```python
from build123d import *

# Parameters (mm, degrees)
ESQUISSE4_R                = 1.3
FIXINGHOLE_DEPTH           = 35
FIXINGHOLEREPETITION_COUNT = 8
RIGHTFIXING_DEPTH          = 10
ESQUISSE7_R                = 1.6
TOPFIXINGHOLES_DEPTH       = 8.6
HOLEFORFIXING_DEPTH        = 51


with BuildPart() as part:
    # Esquisse1 → Révolution1 (revolve)
    with BuildSketch(Plane.XY):
        Polygon((14, 0), (14, 34), (19, 34), (19, 5), (24, 5), (24, 0), align=None)
    revolve(axis=Axis((0, -1.825, 0), (0, 1, 0)))

    # Esquisse4 → FixingHole (cut, through all)
    with BuildSketch(Plane(origin=(0, 0, 0), x_dir=(-1, 0, 0), z_dir=(0, -1, 0))):
        with Locations((0, -22)):
            Circle(ESQUISSE4_R)
    fixinghole = extrude(amount=-FIXINGHOLE_DEPTH, mode=Mode.SUBTRACT)

    # FixingHoleRepetition: FixingHole ×8 about axis
    fixingholerepetition_axis = Axis((0, 0, 0), (0, 1, 0))
    for i in range(1, FIXINGHOLEREPETITION_COUNT):
        add(fixinghole.rotate(fixingholerepetition_axis, i * 360 / FIXINGHOLEREPETITION_COUNT), mode=Mode.SUBTRACT)

    # Esquisse5 → RightFixing (add)
    with BuildSketch(Plane.XY.offset(15)):
        Polygon((9.961946981, 31.674619421), (11.53075035, 13.743114855), (-8.393143611, 12), (-9.961946981, 29.931504566), align=None)
        Polygon((5.40803663, 26.357486686), (5.721797304, 22.771185773), (4.724085983, 22.683897343), (4.976837637, 19.794932719), (5.974548958, 19.882221149), (6.288309632, 16.295920235), (2.702008719, 15.982159562), (2.614720288, 16.979870883), (-0.274244336, 16.727119229), (-0.186955906, 15.729407908), (-3.773256819, 15.415647234), (-4.087017493, 19.001948147), (-3.089306172, 19.089236577), (-3.342057826, 21.978201201), (-4.339769147, 21.890912771), (-4.653529821, 25.477213684), (-1.067228908, 25.790974358), (-0.979940478, 24.793263037), (1.909024147, 25.046014691), (1.821735717, 26.043726012), align=None, mode=Mode.SUBTRACT)
    rightfixing = extrude(amount=RIGHTFIXING_DEPTH)

    # Esquisse7 → TopFixingHoles (cut)
    with BuildSketch(Plane(origin=(12.636394772, 1.10554129, 0), x_dir=(0, 0, -1), z_dir=(0.996194698, 0.087155743, 0))):
        with Locations((-20, 20.835847043)):
            Circle(ESQUISSE7_R)
    topfixingholes = extrude(amount=-TOPFIXINGHOLES_DEPTH, mode=Mode.SUBTRACT)

    # FixingSymetry: RightFixing, TopFixingHoles across plane
    add(rightfixing.mirror(Plane.XY))
    add(topfixingholes.mirror(Plane.XY), mode=Mode.SUBTRACT)

    # Esquisse6 → HoleForFixing (cut, through all)
    with BuildSketch(Plane.XY.offset(25)):
        Polygon((5.40803663, 26.357486686), (5.721797304, 22.771185773), (4.724085983, 22.683897343), (4.976837637, 19.794932719), (5.974548958, 19.882221149), (6.288309632, 16.295920235), (2.702008719, 15.982159562), (2.614720288, 16.979870883), (-0.274244336, 16.727119229), (-0.186955906, 15.729407908), (-3.773256819, 15.415647234), (-4.087017493, 19.001948147), (-3.089306172, 19.089236577), (-3.342057826, 21.978201201), (-4.339769147, 21.890912771), (-4.653529821, 25.477213684), (-1.067228908, 25.790974358), (-0.979940478, 24.793263037), (1.909024147, 25.046014691), (1.821735717, 26.043726012), align=None)
    extrude(amount=-HOLEFORFIXING_DEPTH, mode=Mode.SUBTRACT)


solid = part.part
```
Model file for the job. Use its own axes, mm. A direction names the side the tool comes from. Coordinates: 2 decimals unless noted, no trailing zeros. Loops run counter-clockwise (first coordinate to the right, second up) from the corner with the lowest first, then second, coordinate; pieces in that order, holes last. Notation, with made-up numbers: (74.5, 72) - (112.5, 72) arc R23 ccw to (112.5, 103) - close; hole circle Ø4 at (62.25, 10). An arc over 180 degrees is marked (long way). Write item = value, one per line. Start each with the question number.
Item 1: Saw through at C-C, the plane x = 22. List the corners of the cut face in (y, z).
Item 2: Saw through at A-A, the plane z = 0. List the corners of the cut face in (x, y).
Item 3: Wall check: probe 1 along X at (y, z) = (2, 0); probe 2 along Z at (x, y) = (-5, 18.5); probe 3 along X at (y, z) = (29.5, 11.5). Give the ranges that are in metal, low to high. Write a range as [from, to].
Item 4: Saw through at B-B, the plane y = 13. List the corners of the cut face in (x, z).
Item 5: Pull direction X, two halves, no side cores. Call faces 1 (the face through (0.444, 24.918, 19.513)), 2 (the face through (5.563, 24.589, -18.803)), 3 (the face through (-9.167, 20.84, 20.528)), 4 (the face through (10.735, 22.834, 22.181)): +X half, -X half, draft (parallel to the pull), parting line (faces both ways), or undercut.
Item 6: Drop flat-ended pins along their axis: pin 1 Ø12 at (y, z) = (3.5, -11.5) entering from -X; pin 2 Ø3.5 at (x, z) = (-22, 0) entering from +Y; pin 3 Ø8 at (y, z) = (24.5, 10) entering from +X. Give the stop position or say it passes through.
Item 7: 3-axis set-ups, long thin cutter, end or side, ignore diameter. For faces 5 (the face through (0.28, 2.46, 23.27)), 6 (the face through (-18.98, 19.3, -0.84)), 7 (the face through (-2.89, 25.63, -19.02)), 8 (the face through (-23.27, 2.46, 0.28)), 9 (the face through (1, 26, 25)): which of +Z, -Z, +X, -X, +Y, -Y reach the whole face in a straight line?
Item 8: Saw through at D-D, the plane y = 4. State how many separate pieces and enclosed holes the cut face has, then the cut area to 3 significant figures.
Answers:
q1.outline = (0, -9.59) - (5, -9.59) - (5, -1.3) - (0, -1.3) - close; (0, 1.3) - (5, 1.3) - (5, 9.59) - (0, 9.59) - close
q2.outline = (-24, 0) - (-23.3, 0) - (-23.3, 5) - (-24, 5) - close; (-20.7, 0) - (-14, 0) - (-14, 34) - (-19, 34) - (-19, 5) - (-20.7, 5) - close; (14, 0) - (20.7, 0) - (20.7, 5) - (19, 5) - (19, 34) - (14, 34) - close; (23.3, 0) - (24, 0) - (24, 5) - (23.3, 5) - close
q3.probe_1 = [-24, -23.3], [-20.7, -14], [14, 20.7], [23.3, 24]
q3.probe_2 = [-25, -13.08], [13.08, 25]
q3.probe_3 = [-15.12, -7.98], [7.98, 15.12]
q4.outline = (-8.48, -25) - (3.04, -25) - (3.04, -18.76) arc R19 ccw to (3.04, 18.76) - (3.04, 25) - (-8.48, 25) - (-8.48, 17) arc R19 ccw to (-8.48, -17) - close; hole circle Ø28 at (0, 0)
q5.face_1 = undercut
q5.face_2 = undercut
q5.face_3 = -X half
q5.face_4 = +X half
q6.pin_1 = -23.36
q6.pin_2 = 5
q6.pin_3 = 18.03
q7.face_5 = -Y
q7.face_6 = none
q7.face_7 = +Z, -Z
q7.face_8 = +Y, -Y
q7.face_9 = +Z, +X, -X, +Y, -Y
q8.separate_pieces = 1
q8.enclosed_holes = 9
q8.area = 1,150 mm2
